Read the model definition and answer for the solid it produces. Units are mm, in the model's axes. Face numbers are marked on the shaded views. Coordinates: 2 decimals unless noted, no trailing zeros. Write each loop counter-clockwise with the first axis right and the second up, starting at its lowest first coordinate (ties: lowest second). Pieces come first, ordered by that corner, then holes.
(1) Section B-B on y = 1.5 is taken. Write down the section's boundary in (x, z).
(2) Section A-A on x = 0 is taken. Write down the section's boundary in (y, z).
(3) Given pin 1 (1.5 mm diameter, centred on x = 1, y = 11, fed in from -Z); pin 2 (3 mm diameter, centred on x = 0.5, z = 1, fed in from -Y); pin 3 (1.5 mm diameter, centred on x = 2, y = 7.5, fed in from -Z); pin 4 (0.8 mm diameter, centred on x = 1, y = 16, fed in from +Z), each flat-ended and moving along its own axis, determine where each tip first touches the part or whether it passes through.
(4) Find the intervals of material crossed by probe 1 along Y at (x, z) = (-0.4, 0.4); probe 2 along Z at (x, y) = (0, 0.5); probe 3 along X at (y, z) = (13, 0.25), in increasing order.
(5) The mould has two halves that part along Y. Classify the marked faces 1, 2 and 3: +Y half, -Y half, draft (parallel to the pull), parting line (faces both ways), or undercut.
(6) Section C-C on z = 0 is taken. Write down the section's boundary in (x, y), then the cut area to 4 significant figures.
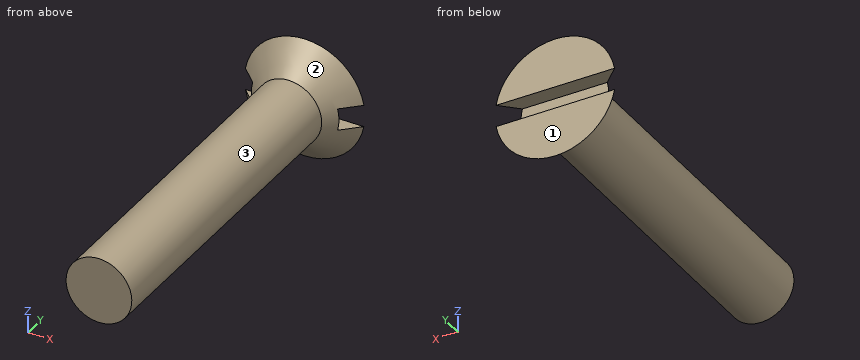
from build123d import *

# Parameters (mm, degrees)
SKETCH2_W          = 5.5
SKETCH2_H          = 1
CUT_EXTRUDE1_DEPTH = 0.75


with BuildPart() as part:
    # Sketch1 → Revolve1 (revolve)
    with BuildSketch(Plane(origin=(0, 0, 0), x_dir=(0, 0, -1), z_dir=(1, 0, 0))):
        Polygon((0, 0), (-1.5, 0), (-1.5, 15), (-2.75, 16.25), (0, 16.25), align=None)
    revolve(axis=Axis((0, 16.25, 0), (0, -1, 0)))

    # Sketch2 → Cut-Extrude1 (cut)
    with BuildSketch(Plane(origin=(0, 16.25, 0), x_dir=(1, 0, 0), z_dir=(0, 1, 0))):
        Rectangle(SKETCH2_W, SKETCH2_H)
    extrude(amount=-CUT_EXTRUDE1_DEPTH, mode=Mode.SUBTRACT)


solid = part.part
Response:
1. outline: circle Ø3 at (0, 0)
2. outline: (0, -1.5) - (15, -1.5) - (16.25, -2.75) - (16.25, -0.5) - (15.5, -0.5) - (15.5, 0.5) - (16.25, 0.5) - (16.25, 2.75) - (15, 1.5) - (0, 1.5) - close
3. pin 1: stops at z = -1.48
3. pin 2: stops at y = 0
3. pin 3: stops at z = -0.83
3. pin 4: stops at z = 2.66
4. probe 1: y = 0 to 15.5
4. probe 2: z = -1.5 to 1.5
4. probe 3: x = -1.48 to 1.48
5. face 1: +Y half
5. face 2: -Y half
5. face 3: draft
6. outline: (-2, 15.5) - (-1.5, 15) - (-1.5, 0) - (1.5, 0) - (1.5, 15) - (2, 15.5) - close
6. area: 46.75 mm2
